```python
from build123d import *
from build123d.topology import SkipClean

# Parameters (mm, degrees)
DODANIE_WYCI_GNI_CIE1_DEPTH = 2
SZKIC_START                 = -28.065385
SZKIC_ZGI_CIA1_DEPTH        = 54
SZKIC_ZGI_CIA1_2_DEPTH      = 15.5
SZKIC_START_2               = 10.434615
SZKIC_ZGI_CIA1_3_DEPTH      = 15.5
SZKIC_START_3               = -56.031828
SZKIC_ZGI_CIA1_4_DEPTH      = 2.423909
SZKIC_START_4               = -12.565385
SZKIC_ZGI_CIA1_5_DEPTH      = 23
SZKIC_ZGI_CIA1_6_DEPTH      = 23
SZKIC_ZGI_CIA2_DEPTH        = 54
SZKIC_ZGI_CIA2_2_DEPTH      = 54
SZKIC_START_5               = 49.968172
SZKIC_ZGI_CIA2_3_DEPTH      = 2
SZKIC9_W                    = 72
SZKIC9_H                    = 28
SZKIC9_W_2                  = 15
SZKIC9_H_2                  = 7
WYTNIJ_WYCI_GNI_CIE1_DEPTH  = 66.825561
SZKIC10_R                   = 1.5
WYTNIJ_WYCI_GNI_CIE2_DEPTH  = 114.762973
ZAOKR_GLENIE2_R             = 1
ZAOKR_GLENIE3_R             = 1


with BuildPart() as part:
    # Szkic1 → Dodanie-wyciągnięcie1 (new body)
    with BuildSketch(Plane.XY):
        with BuildLine():
            Line((-75.531828, 25.934615), (71.468172, 25.934615))
            Line((71.468172, 25.934615), (71.468172, 10.434615))
            ThreePointArc((71.468172, 10.434615), (59.968172, -1.065385), (71.468172, -12.565385))
            Line((71.468172, -12.565385), (71.468172, -28.065385))
            Line((71.468172, -28.065385), (-75.531828, -28.065385))
            Line((-75.531828, -28.065385), (-75.531828, -12.565385))
            ThreePointArc((-75.531828, -12.565385), (-64.031828, -1.065385), (-75.531828, 10.434615))
            Line((-75.531828, 10.434615), (-75.531828, 25.934615))
        make_face()
    extrude(amount=DODANIE_WYCI_GNI_CIE1_DEPTH)

    # Szkic zgięcia1: read off the stored shape, not the designer's step
    # Szkic zgięcia1 outline → Szkic zgięcia1 (cut)
    with BuildSketch(Plane(origin=(0, 0, 0), x_dir=(1, 0, 0), z_dir=(0, 1, 0)).offset(SZKIC_START)):
        with BuildLine():
            Line((-75.531828, -2), (-55.981318, -2))
            ThreePointArc((-55.981318, -2), (-55.112967, -0.563508), (-53.531828, 0))
            Line((-53.531828, 0), (-75.531828, 0))
            Line((-75.531828, 0), (-75.531828, -2))
        make_face()
    extrude(amount=SZKIC_ZGI_CIA1_DEPTH, mode=Mode.SUBTRACT)

    # Szkic zgi_cia1 2 outline → Szkic zgi_cia1 2 (add)
    with BuildSketch(Plane(origin=(0, 0, 0), x_dir=(1, 0, 0), z_dir=(0, 1, 0)).offset(SZKIC_START)):
        with BuildLine():
            ThreePointArc((-55.981318, -2), (-56.019168, -2.248728), (-56.031828, -2.5))
            Line((-56.031828, -2.5), (-56.031828, -22.143806))
            Line((-56.031828, -22.143806), (-54.031828, -22.143806))
            Line((-54.031828, -22.143806), (-54.031828, -2.5))
            ThreePointArc((-54.031828, -2.5), (-53.885381, -2.146447), (-53.531828, -2))
            Line((-53.531828, -2), (-55.981318, -2))
        make_face()
    extrude(amount=SZKIC_ZGI_CIA1_2_DEPTH)

    # Szkic zgi_cia1 3 outline → Szkic zgi_cia1 3 (add)
    with BuildSketch(Plane(origin=(0, 0, 0), x_dir=(1, 0, 0), z_dir=(0, 1, 0)).offset(SZKIC_START_2)):
        with BuildLine():
            ThreePointArc((-55.981318, -2), (-56.019168, -2.248728), (-56.031828, -2.5))
            Line((-56.031828, -2.5), (-56.031828, -22.143806))
            Line((-56.031828, -22.143806), (-54.031828, -22.143806))
            Line((-54.031828, -22.143806), (-54.031828, -2.5))
            ThreePointArc((-54.031828, -2.5), (-53.885381, -2.146447), (-53.531828, -2))
            Line((-53.531828, -2), (-55.981318, -2))
        make_face()
    extrude(amount=SZKIC_ZGI_CIA1_3_DEPTH)

    # Szkic zgi_cia1 4 outline → Szkic zgi_cia1 4 (add)
    with BuildSketch(Plane.YZ.offset(SZKIC_START_3)):
        with BuildLine():
            Line((10.434615, 2), (10.434615, 22.143806))
            ThreePointArc((10.434615, 22.143806), (-1.065385, 10.643806), (-12.565385, 22.143806))
            Line((-12.565385, 22.143806), (-12.565385, 2))
            Line((-12.565385, 2), (10.434615, 2))
        make_face()
    extrude(amount=SZKIC_ZGI_CIA1_4_DEPTH)

    # Szkic zgi_cia1 5 outline → Szkic zgi_cia1 5 (cut)
    with SkipClean():  # the faces are left unmerged after this step: merging them gives an invalid solid
        with BuildSketch(Plane(origin=(0, 0, 0), x_dir=(1, 0, 0), z_dir=(0, 1, 0)).offset(SZKIC_START_4)):
            with BuildLine():
                ThreePointArc((-53.607919, -2.005824), (-53.911331, -2.174459), (-54.031828, -2.5))
                Line((-54.031828, -2.5), (-54.031828, -24))
                Line((-54.031828, -24), (-53.607919, -24))
                Line((-53.607919, -24), (-53.607919, -2.005824))
            make_face()
            with BuildLine():
                Line((-58, -24), (-56.031828, -24))
                Line((-56.031828, -24), (-56.031828, -2.5))
                ThreePointArc((-56.031828, -2.5), (-56.019168, -2.248728), (-55.981318, -2))
                Line((-55.981318, -2), (-58, -2))
                Line((-58, -2), (-58, -24))
            make_face()
        extrude(amount=SZKIC_ZGI_CIA1_5_DEPTH, mode=Mode.SUBTRACT)

    # Szkic zgi_cia1 6 outline → Szkic zgi_cia1 6 (add)
    with SkipClean():  # the faces are left unmerged after this step: merging them gives an invalid solid
        with BuildSketch(Plane(origin=(0, 0, 0), x_dir=(1, 0, 0), z_dir=(0, 1, 0)).offset(SZKIC_START_4)):
            with BuildLine():
                Line((-53.607919, -2), (-53.607919, -2.005824))
                ThreePointArc((-53.607919, -2.005824), (-53.569985, -2.001458), (-53.531828, -2))
                Line((-53.531828, -2), (-53.607919, -2))
            make_face()
        extrude(amount=SZKIC_ZGI_CIA1_6_DEPTH)

    # Szkic zgięcia2: read off the stored shape, not the designer's step
    # Szkic zgięcia2 outline → Szkic zgięcia2 (cut)
    with SkipClean():  # the faces are left unmerged after this step: merging them gives an invalid solid
        with BuildSketch(Plane(origin=(0, 0, 0), x_dir=(1, 0, 0), z_dir=(0, 1, 0)).offset(SZKIC_START)):
            with BuildLine():
                ThreePointArc((49.468172, 0), (51.049311, -0.563508), (51.917662, -2))
                Line((51.917662, -2), (71.468172, -2))
                Line((71.468172, -2), (71.468172, 0))
                Line((71.468172, 0), (49.468172, 0))
            make_face()
        extrude(amount=SZKIC_ZGI_CIA2_DEPTH, mode=Mode.SUBTRACT)

    # Szkic zgi_cia2 2 outline → Szkic zgi_cia2 2 (add)
    with SkipClean():  # the faces are left unmerged after this step: merging them gives an invalid solid
        with BuildSketch(Plane(origin=(0, 0, 0), x_dir=(1, 0, 0), z_dir=(0, 1, 0)).offset(SZKIC_START)):
            with BuildLine():
                Line((49.968172, -22.143806), (51.968172, -22.143806))
                Line((51.968172, -22.143806), (51.968172, -2.5))
                ThreePointArc((51.968172, -2.5), (51.955512, -2.248728), (51.917662, -2))
                Line((51.917662, -2), (49.468172, -2))
                ThreePointArc((49.468172, -2), (49.821725, -2.146447), (49.968172, -2.5))
                Line((49.968172, -2.5), (49.968172, -22.143806))
            make_face()
        extrude(amount=SZKIC_ZGI_CIA2_2_DEPTH)

    # Szkic zgi_cia2 3 outline → Szkic zgi_cia2 3 (cut)
    with SkipClean():  # the faces are left unmerged after this step: merging them gives an invalid solid
        with BuildSketch(Plane.YZ.offset(SZKIC_START_5)):
            with BuildLine():
                Line((10.434615, 22.143806), (-12.565385, 22.143806))
                ThreePointArc((-12.565385, 22.143806), (-1.065385, 10.643806), (10.434615, 22.143806))
            make_face()
        extrude(amount=SZKIC_ZGI_CIA2_3_DEPTH, mode=Mode.SUBTRACT)

    # Szkic9 → Wytnij-wyciągnięcie1 (cut, through all)
    with SkipClean():  # the faces are left unmerged after this step: merging them gives an invalid solid
        with BuildSketch(Plane.XY.offset(2)):
            with Locations((-8.031828, -1.065385)):
                Rectangle(SZKIC9_W, SZKIC9_H)
            with Locations((35.468172, 22.434615)):
                Rectangle(SZKIC9_W_2, SZKIC9_H_2)
            with BuildLine():
                Line((-9.515655, 18.934615), (5.451999, 18.934615))
                ThreePointArc((5.451999, 18.934615), (6.451999, 17.934615), (5.451999, 16.934615))
                Line((5.451999, 16.934615), (-9.515655, 16.934615))
                ThreePointArc((-9.515655, 16.934615), (-10.515655, 17.934615), (-9.515655, 18.934615))
            make_face()
            with BuildLine():
                Line((-9.515655, -19.065385), (5.451999, -19.065385))
                ThreePointArc((5.451999, -19.065385), (6.451999, -20.065385), (5.451999, -21.065385))
                Line((5.451999, -21.065385), (-9.515655, -21.065385))
                ThreePointArc((-9.515655, -21.065385), (-10.515655, -20.065385), (-9.515655, -19.065385))
            make_face()
        extrude(amount=-WYTNIJ_WYCI_GNI_CIE1_DEPTH, mode=Mode.SUBTRACT)

    # Szkic10 → Wytnij-wyciągnięcie2 (cut, through all)
    with SkipClean():  # the faces are left unmerged after this step: merging them gives an invalid solid
        with BuildSketch(Plane.ZY.offset(56.031828)):
            with Locations((7.643806, 14.434615)):
                Circle(SZKIC10_R)
            with Locations((7.643806, -16.565385)):
                Circle(SZKIC10_R)
        extrude(amount=-WYTNIJ_WYCI_GNI_CIE2_DEPTH, mode=Mode.SUBTRACT)

    # Zaokrąglenie2
    zaokr_glenie2_edges = [part.edges().sort_by_distance(p)[0] for p in [
        (27.968172, 25.934615, 1),
        (42.968172, 25.934615, 1),
    ]]
    fillet(zaokr_glenie2_edges, radius=ZAOKR_GLENIE2_R)

    # Zaokrąglenie3
    zaokr_glenie3_edges = [part.edges().sort_by_distance(p)[0] for p in [
        (-44.031828, -15.065385, 1),
        (-44.031828, 12.934615, 1),
        (27.968172, 12.934615, 1),
        (27.968172, -15.065385, 1),
    ]]
    fillet(zaokr_glenie3_edges, radius=ZAOKR_GLENIE3_R)


solid = part.part
```
Source: CAD feature listing. Evaluate the final solid. Frame: model axes, mm. A direction names the side the tool comes from. Round coordinates to 2 decimals unless told otherwise and drop trailing zeros. Order: outer loops, then holes, each group sorted by start corner. A loop starts at its lowest first (then second) coordinate and runs counter-clockwise, first axis right, second up. Notation, with made-up numbers: (58, 85.5) -> (68, 85.5) arc R22 cw to (68, 120.5) -> close; hole circle Ø7 at (67, 49.5). An arc over 180 degrees is marked (long way). Use CSV: the item, a comma, the result in double quotes.
(1) Section B-B on z = 3.5. Return the cut outline in (x, y), and give its area (3 significant figures).
Report:
outline,"(-56.03, -28.07) -> (-54.03, -28.07) -> (-54.03, 25.93) -> (-56.03, 25.93) -> close; (49.97, -28.07) -> (51.97, -28.07) -> (51.97, 25.93) -> (49.97, 25.93) -> close"
area,"216 mm^2"
(2) First-contact query: pin 1 Ø6 at (x, y) = (-34, -15) entering from +Z; pin 2 Ø1 at (y, z) = (21.5, 1) entering from -X; pin 3 Ø0.6 at (x, z) = (36.5, 1) entering from +Y. Flat tips, straight axial feed; report the tip coordinate or a pass-through.
Report:
pin 1,"z = 2"
pin 2,"x = -55.82"
pin 3,"y = 18.93"
(3) Ray query, L1, parallel to X at y = 9.5, z = 2.5; L2, parallel to Z at x = 17.5, y = 19. Return the intervals inside material, ascending.
Report:
L1,"-56.03 to -54.03, 49.97 to 51.97"
L2,"0 to 2"
(4) Section C-C on y = 21.5. Return the cut outline in (x, z), and give its area (3 significant figures).
Report:
outline,"(-56.03, 2.5) arc R2.5 ccw to (-55.98, 2) arc R2.5 ccw to (-53.53, 0) -> (27.97, 0) -> (27.97, 2) -> (-53.53, 2) arc R0.5 cw to (-54.03, 2.5) -> (-54.03, 22.14) -> (-56.03, 22.14) -> close; (42.97, 0) -> (49.47, 0) arc R2.5 ccw to (51.92, 2) arc R2.5 ccw to (51.97, 2.5) -> (51.97, 22.14) -> (49.97, 22.14) -> (49.97, 2.5) arc R0.5 cw to (49.47, 2) -> (42.97, 2) -> close"
area,"264 mm^2"
(5) Pull-direction query (Y, two-part tool) for faces 4 (the face through (-55, 18, 22.144)), 5 (the face through (-55.046, -0.813, 10.647)); classes: +Y half, -Y half, draft (parallel to the pull), parting line (faces both ways), or undercut.
Report:
face 4,"draft"
face 5,"undercut"
(6) Section D-D on x = -32. Return the cut outline in (y, z), and give its area (3 significant figures).
Report:
outline,"(-28.07, 0) -> (-15.07, 0) -> (-15.07, 2) -> (-28.07, 2) -> close; (12.93, 0) -> (25.93, 0) -> (25.93, 2) -> (12.93, 2) -> close"
area,"52.0 mm^2"
(7) Section A-A on x = 4. Return the cut outline in (y, z).
Report:
outline,"(-28.07, 0) -> (-21.07, 0) -> (-21.07, 2) -> (-28.07, 2) -> close; (-19.07, 0) -> (-15.07, 0) -> (-15.07, 2) -> (-19.07, 2) -> close; (12.93, 0) -> (16.93, 0) -> (16.93, 2) -> (12.93, 2) -> close; (18.93, 0) -> (25.93, 0) -> (25.93, 2) -> (18.93, 2) -> close"
(8) Access query for faces 1 (the face through (27.968, 22, 1)), 2 (the face through (-2, -21.065, 1)), 3 (the face through (-54.032, -1, 10)). Directions: +Z, -Z, +X, -X, +Y, -Y. A direction counts if a zero-diameter tool reaches every point of the face in a straight line with its end or side. Return the directions, or none.
Report:
face 1,"+Z, -Z, +Y"
face 2,"+Z, -Z"
face 3,"+Z, +Y, -Y"
